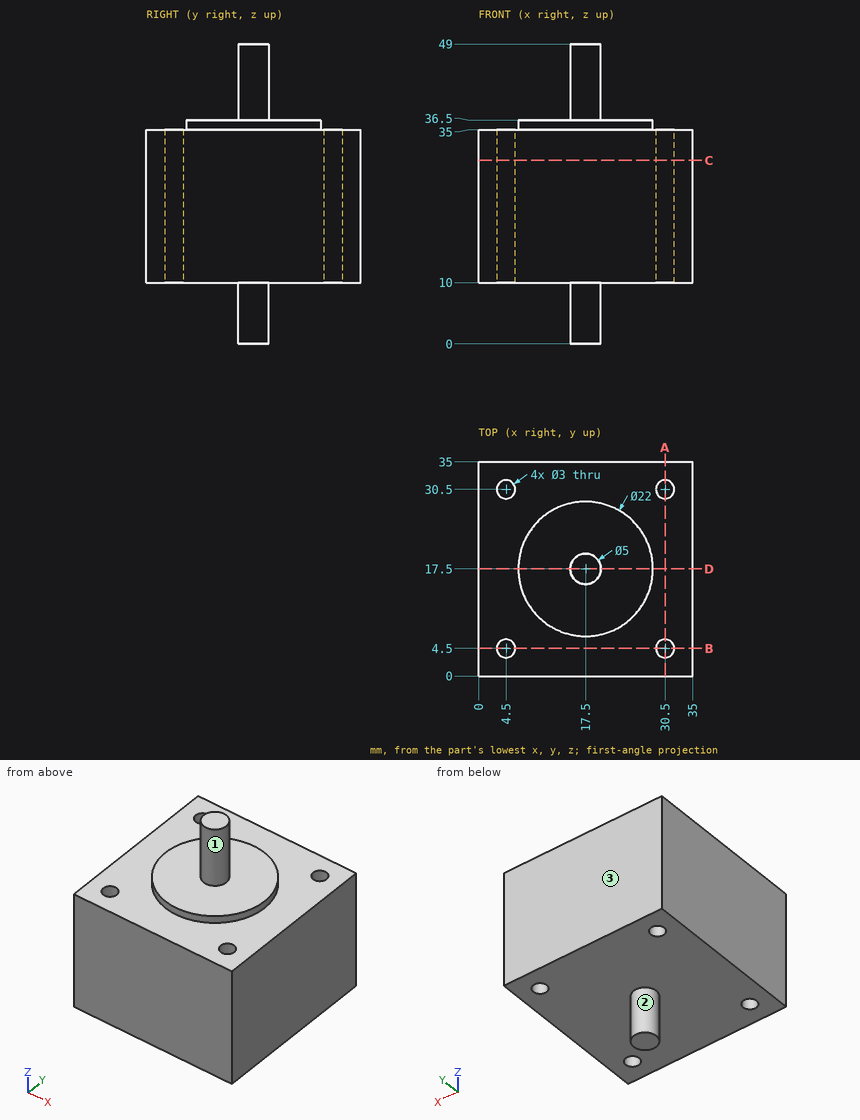
Answer from the drawing. Dimensions are ordinates in mm from the lowest x, y and z of the part. A direction names the side the tool comes from. Give positions to 0.01 mm unless a question says otherwise; leave off trailing zeros. Order: outer loops, then holes, each group sorted by start corner. A loop starts at its lowest first (then second) coordinate and runs counter-clockwise, first axis right, second up. Notation, with made-up numbers: (26.5, 12) -> (83.5, 12) arc R19 cw to (83.5, 41) -> close; hole circle Ø4 at (57.25, -4.5). An arc over 180 degrees is marked (long way). One line per item, written item: value.
Item 1: A tool of negligible diameter and unlimited length cuts with its end or side. For the marked faces 1, 2 and 3, from which of +Z, -Z, +X, -X, +Y, -Y can it reach the whole face along a straight path? Write none if from no direction.
Answer sheet:
face 1: +Z
face 2: -Z
face 3: +Z, -Z, +X, -X, +Y
Item 2: Straight lines are drawn through the part: probe 1 along Y at (x, z) = (4.5, 22.5); probe 2 along Z at (x, y) = (7, 28); probe 3 along X at (y, z) = (4, 25). For each, find the intervals that lie inside material, in ascending order.
Answer sheet:
probe 1: 0 to 3, 6 to 29, 32 to 35
probe 2: 10 to 35
probe 3: 0 to 3.09, 5.91 to 29.09, 31.91 to 35
Item 3: Find section C-C, the plane z = 30. Give the vertices of the cut face in (x, y), plus the area to 3 significant figures.
Answer sheet:
outline: (0, 0) -> (35, 0) -> (35, 35) -> (0, 35) -> close; hole circle Ø3 at (4.5, 4.5); hole circle Ø3 at (4.5, 30.5); hole circle Ø3 at (30.5, 4.5); hole circle Ø3 at (30.5, 30.5)
area: 1,200 mm²
Item 4: Find section D-D, the plane y = 17.5. Give the vertices of the cut face in (x, z).
Answer sheet:
outline: (0, 10) -> (15, 10) -> (15, 0) -> (20, 0) -> (20, 10) -> (35, 10) -> (35, 35) -> (28.5, 35) -> (28.5, 36.5) -> (20, 36.5) -> (20, 49) -> (15, 49) -> (15, 36.5) -> (6.5, 36.5) -> (6.5, 35) -> (0, 35) -> close
Item 5: Flat-ended cylindrical pins translate along their axes: P1, Ø2.5, axis at x = 4.5, y = 4.5, coming from the +Z side; P2, Ø1, axis at x = 6, y = 5.5, coming from the +Z side; P3, Ø10, axis at x = 16, z = 5.5, coming from the +Y side; P4, Ø2, axis at x = 5.5, y = 4.5, coming from the -Z side. Find the tip coordinate at first contact, or state that the pin passes through.
Answer sheet:
P1: through
P2: z = 35
P3: y = 35
P4: z = 10
Item 6: Find section A-A, the plane x = 30.5. Give the vertices of the cut face in (y, z), plus the area to 3 significant figures.
Answer sheet:
outline: (0, 10) -> (3, 10) -> (3, 35) -> (0, 35) -> close; (6, 10) -> (29, 10) -> (29, 35) -> (6, 35) -> close; (32, 10) -> (35, 10) -> (35, 35) -> (32, 35) -> close
area: 725 mm²
